from build123d import *

# Parameters (mm, degrees)
SKETCH1_W           = 23
SKETCH1_H           = 60
BOSS_EXTRUDE1_DEPTH = 4
SKETCH2_W           = 19
SKETCH2_H           = 3.65261657
CUT_EXTRUDE1_DEPTH  = 65.399961729
SKETCH4_R           = 2
CUT_EXTRUDE2_DEPTH  = 103.729507508


with BuildPart() as part:
    # Sketch1 → Boss-Extrude1 (new body)
    with BuildSketch(Plane.XY):
        with Locations((11.551140333, -70.029978717)):
            Rectangle(SKETCH1_W, SKETCH1_H)
    extrude(amount=BOSS_EXTRUDE1_DEPTH)

    # Sketch2 → Cut-Extrude1 (cut, through all)
    with BuildSketch(Plane(origin=(0, -40.029978717, 0), x_dir=(1, 0, 0), z_dir=(0, 1, 0))):
        with Locations((11.551140333, -2.826308285)):
            Rectangle(SKETCH2_W, SKETCH2_H)
    extrude(amount=-CUT_EXTRUDE1_DEPTH, mode=Mode.SUBTRACT)

    # Sketch4 → Cut-Extrude2 (cut, through all)
    with BuildSketch(Plane(origin=(0, 0, 0), x_dir=(-1, 0, 0), z_dir=(0, 0, -1))):
        with Locations((-11.551140333, -50.029978717)):
            Circle(SKETCH4_R)
        with Locations((-11.551140333, -90.029978717)):
            Circle(SKETCH4_R)
    extrude(amount=-CUT_EXTRUDE2_DEPTH, mode=Mode.SUBTRACT)


solid = part.part
Part model, mm, in its own coordinate system. A direction names the side the tool comes from. Round coordinates to 2 decimals unless told otherwise and drop trailing zeros. Order: outer loops, then holes, each group sorted by start corner. A loop starts at its lowest first (then second) coordinate and runs counter-clockwise, first axis right, second up. Notation, with made-up numbers: (82.25, 15.25) -> (88.25, 15.25) arc R20 ccw to (88.25, 43.25) -> close; hole circle Ø10 at (-4, -35). An arc over 180 degrees is marked (long way). Put each result on its own line as item: value.
Q1. Wall check: line 1 (X direction, y = -85, z = 2.6); line 2 (Y direction, x = 9.75, z = 0.65); line 3 (Z direction, x = 17, y = -82). Give the ranges that are in metal, low to high. Write a range as [from, to].
From the geometry:
line 1: x = [0.05, 2.05], [21.05, 23.05]
line 2: y = [-100.03, -90.9], [-89.16, -50.9], [-49.16, -40.03]
line 3: z = [0, 1]
Q2. Pin check, flat tip, straight feed: pin 1 Ø5 at (x, y) = (11.55, -50.03) entering from +Z. Stop position of the tip, or through.
From the geometry:
pin 1: stops at z = 1
Q3. Band-saw the part on D-D (x = 15.75). Give the cut face in (y, z).
From the geometry:
outline: (-100.03, 0) -> (-40.03, 0) -> (-40.03, 1) -> (-100.03, 1) -> close
Q4. Band-saw the part on A-A (z = 3.25). Give the cut face in (x, y), and give its area (3 significant figures).
From the geometry:
outline: (0.05, -100.03) -> (2.05, -100.03) -> (2.05, -40.03) -> (0.05, -40.03) -> close; (21.05, -100.03) -> (23.05, -100.03) -> (23.05, -40.03) -> (21.05, -40.03) -> close
area: 240 mm2
Q5. Band-saw the part on C-C (x = 10.5). Give the cut face in (y, z).
From the geometry:
outline: (-100.03, 0) -> (-91.73, 0) -> (-91.73, 1) -> (-100.03, 1) -> close; (-88.33, 0) -> (-51.73, 0) -> (-51.73, 1) -> (-88.33, 1) -> close; (-48.33, 0) -> (-40.03, 0) -> (-40.03, 1) -> (-48.33, 1) -> close
Q6. Tool access for faces 1 (the face through (1, -70, 4)), 2 (the face through (2.051, -70, 3)): list every direction of +Z, -Z, +X, -X, +Y, -Y with a clear straight run to the whole face (end or side of a thin tool).
From the geometry:
face 1: +Z, +X, -X, +Y, -Y
face 2: +Z, +Y, -Y
Q7. Band-saw the part on B-B (y = -79.5). Give the cut face in (x, z).
From the geometry:
outline: (0.05, 0) -> (23.05, 0) -> (23.05, 4) -> (21.05, 4) -> (21.05, 1) -> (2.05, 1) -> (2.05, 4) -> (0.05, 4) -> close
